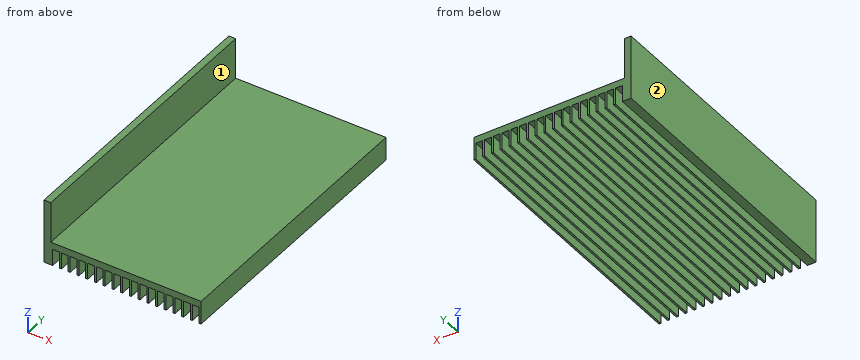
Autodesk Inventor part; units mm, degrees
ref_plane "YZ Plane" through (0, 0, 0) normal (1, 0, 0) x (0, 1, 0)
ref_plane "XZ Plane" through (0, 0, 0) normal (0, 1, 0) x (-1, 0, 0)
ref_plane "XY Plane" through (0, 0, 0) normal (0, 0, 1) x (1, 0, 0)
sketch "Skizze1" plane through (0, 0, 0) normal (0, 0, 1) x (1, 0, 0)
  line L0 (-40.5, -71.5) -> (40.5, -71.5)
  line L1 (40.5, -71.5) -> (40.5, 71.5)
  line L2 (40.5, 71.5) -> (-40.5, 71.5)
  line L3 (-40.5, 71.5) -> (-40.5, -71.5)
  line L4 (-40.5, -71.5) -> (40.5, 71.5) construction
  line L5 (40.5, -71.5) -> (-40.5, 71.5) construction
  point P0 (0, 0)
  dimension "d0" = 143
  dimension "d1" = 81
extrude "Grundkörper" add sketch "Skizze1" along normal blind 33
sketch "Skizze2" plane through (-40.5, -71.5, 0) normal (0, -1, 0) x (1, 0, 0)
  line L0 (0, 0) -> (0, 33)
  line L1 (0, 0) -> (81, 0)
  line L2 (0, 0) -> (81, 0)
  line L3 (81, 0) -> (81, 33)
  line L4 (0, 33) -> (81, 33)
  line L5 (0, 0) -> (0, 33)
  line L6 (81, 0) -> (81, 33)
  line L7 (3.5, 33) -> (3.5, 12)
  line L8 (3.5, 12) -> (81, 12)
  point P0 (40.5, 0)
  dimension "d4" = 12
  dimension "d5" = 3.5
extrude "Ausschnitt" cut sketch "Skizze2" against normal through all contours L4 L3 L8 L7
sketch "Skizze3" plane through (-40.5, -71.5, 0) normal (0, -1, 0) x (1, 0, 0)
  line L0 (0, 0) -> (81, 0) construction
  line L1 (81, 0) -> (81, 12) construction
  line L2 (81, 0) -> (0, 0) construction
  line L3 (76.5, 0) -> (80, 0)
  line L4 (80, 0) -> (80, 8.5)
  line L5 (80, 8.5) -> (76.5, 8.5)
  line L6 (76.5, 8.5) -> (76.5, 0)
  line L7 (72, 8.5) -> (72, 0)
  line L8 (72, 0) -> (75.5, 0)
  line L9 (75.5, 0) -> (75.5, 8.5)
  line L10 (75.5, 8.5) -> (72, 8.5)
  line L11 (67.5, 8.5) -> (67.5, 0)
  line L12 (67.5, 0) -> (71, 0)
  line L13 (71, 0) -> (71, 8.5)
  line L14 (71, 8.5) -> (67.5, 8.5)
  line L15 (63, 8.5) -> (63, 0)
  line L16 (63, 0) -> (66.5, 0)
  line L17 (66.5, 0) -> (66.5, 8.5)
  line L18 (66.5, 8.5) -> (63, 8.5)
  line L19 (58.5, 8.5) -> (58.5, 0)
  line L20 (58.5, 0) -> (62, 0)
  line L21 (62, 0) -> (62, 8.5)
  line L22 (62, 8.5) -> (58.5, 8.5)
  line L23 (54, 8.5) -> (54, 0)
  line L24 (54, 0) -> (57.5, 0)
  line L25 (57.5, 0) -> (57.5, 8.5)
  line L26 (57.5, 8.5) -> (54, 8.5)
  line L27 (49.5, 8.5) -> (49.5, 0)
  line L28 (49.5, 0) -> (53, 0)
  line L29 (53, 0) -> (53, 8.5)
  line L30 (53, 8.5) -> (49.5, 8.5)
  line L31 (45, 8.5) -> (45, 0)
  line L32 (45, 0) -> (48.5, 0)
  line L33 (48.5, 0) -> (48.5, 8.5)
  line L34 (48.5, 8.5) -> (45, 8.5)
  line L35 (40.5, 8.5) -> (40.5, 0)
  line L36 (40.5, 0) -> (44, 0)
  line L37 (44, 0) -> (44, 8.5)
  line L38 (44, 8.5) -> (40.5, 8.5)
  line L39 (36, 8.5) -> (36, 0)
  line L40 (36, 0) -> (39.5, 0)
  line L41 (39.5, 0) -> (39.5, 8.5)
  line L42 (39.5, 8.5) -> (36, 8.5)
  line L43 (31.5, 8.5) -> (31.5, 0)
  line L44 (31.5, 0) -> (35, 0)
  line L45 (35, 0) -> (35, 8.5)
  line L46 (35, 8.5) -> (31.5, 8.5)
  line L47 (27, 8.5) -> (27, 0)
  line L48 (27, 0) -> (30.5, 0)
  line L49 (30.5, 0) -> (30.5, 8.5)
  line L50 (30.5, 8.5) -> (27, 8.5)
  line L51 (22.5, 8.5) -> (22.5, 0)
  line L52 (22.5, 0) -> (26, 0)
  line L53 (26, 0) -> (26, 8.5)
  line L54 (26, 8.5) -> (22.5, 8.5)
  line L55 (18, 8.5) -> (18, 0)
  line L56 (18, 0) -> (21.5, 0)
  line L57 (21.5, 0) -> (21.5, 8.5)
  line L58 (21.5, 8.5) -> (18, 8.5)
  line L59 (13.5, 8.5) -> (13.5, 0)
  line L60 (13.5, 0) -> (17, 0)
  line L61 (17, 0) -> (17, 8.5)
  line L62 (17, 8.5) -> (13.5, 8.5)
  line L63 (9, 8.5) -> (9, 0)
  line L64 (9, 0) -> (12.5, 0)
  line L65 (12.5, 0) -> (12.5, 8.5)
  line L66 (12.5, 8.5) -> (9, 8.5)
  line L67 (4.5, 8.5) -> (4.5, 0)
  line L68 (4.5, 0) -> (8, 0)
  line L69 (8, 0) -> (8, 8.5)
  line L70 (8, 8.5) -> (4.5, 8.5)
  point P0 (40.5, 0)
  dimension "d11" = 1
  dimension "d12" = 8.5
  dimension "d13" = 3.5
  dimension "d16" = 4.5
extrude "Kühlrippen" cut sketch "Skizze3" against normal through all
properties part number "800-20-MOTOR-CONTROLLER-BLD-300B-01" material "Aluminium 6061"
Part model, mm, in its own coordinate system. Face numbers are marked on the shaded views. A direction names the side the tool comes from. Round coordinates to 2 decimals unless told otherwise and drop trailing zeros. Write each loop counter-clockwise with the first axis right and the second up, starting at its lowest first coordinate (ties: lowest second). Pieces come first, ordered by that corner, then holes. Notation, with made-up numbers: M -25.5,84.25 L 21.5,84.25 A25 ccw 21.5,105.25 Z; hole C 13.5,25.25 d2. An arc over 180 degrees is marked long. Answer as CSV lines item,"result". Start each with the question number.
1) Drop a flat-ended pin along its axis: pin 1 (1.8 mm diameter, centred on x = -34.5, y = -28, fed in from -Z). Give the stop position or say it passes through.
2) Band-saw the part on C-C (x = -34.5). List the corners of the cut face in (y, z).
3) Drill centre lines: L1, parallel to Z at x = 12, y = 24.5; L2, parallel to X at y = -43.5, z = 13; L3, parallel to Z at x = -18.5, y = 4. Where is each one in solid material? Low to high.
4) Which spindle directions (+Z, -Z, +X, -X, +Y, -Y) get a long thin tool onto all of the face, cutting with end or side? Do the marked faces 1 and 2. Say none if no direction does.
5) Band-saw the part on B-B (z = 25). List the corners of the cut face in (x, y).
6) Band-saw the part on A-A (z = 5.5). Count the separate pieces of the cut face and the enclosed holes in it, then the cut area to 3 significant figures.
Worked out:
1,pin 1,"z = 8.5"
2,outline,"M -71.5,8.5 L 71.5,8.5 L 71.5,12 L -71.5,12 Z"
3,L1,"8.5 to 12"
3,L2,"-40.5 to -37"
3,L3,"0 to 12"
4,face 1,"+Z, +X, +Y, -Y"
4,face 2,"+Z, -Z, -X, +Y, -Y"
5,outline,"M -40.5,-71.5 L -37,-71.5 L -37,71.5 L -40.5,71.5 Z"
6,separate pieces,"18"
6,enclosed holes,"0"
6,area,"3,070 mm²"
